For this review, take the finished solid that the model builds, in its own axes (mm). Face numbers are marked on the shaded views. A direction names the side the tool comes from. Coordinates: 2 decimals unless noted, no trailing zeros. Order: outer loops, then holes, each group sorted by start corner. A loop starts at its lowest first (then second) coordinate and runs counter-clockwise, first axis right, second up.
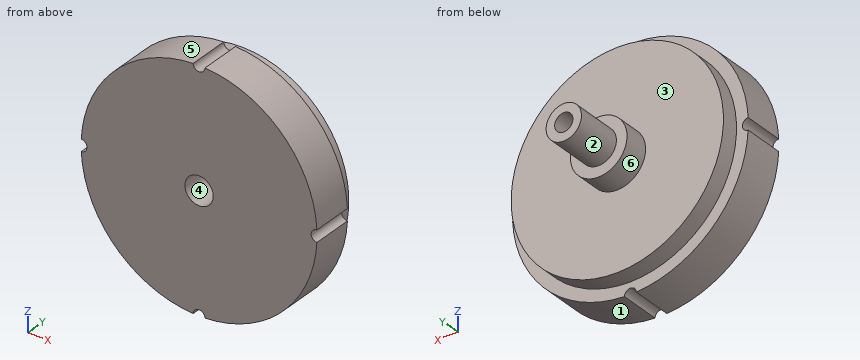
from build123d import *

# Parameters (mm, degrees)
CUT_EXTRUDE1_DEPTH      = 18.993488406
CUT_EXTRUDE1_DEPTH_BACK = 18.993488406
SKETCH5_R               = 0.5


with BuildPart() as part:
    # Sketch4 → Revolve1 (revolve)
    with BuildSketch(Plane.XY, mode=Mode.PRIVATE) as revolve1_sk:
        Polygon((-0.775, 11.125), (-0.775, 4), (-1.2, 4), (-1.2, 0), (-10, 0), (-10, 3.5), (-9, 3.5), (-9, 5), (-2.4, 5), (-2.4, 7.125), (-1.5, 7.125), (-1.5, 11.125), align=None)
    revolve(revolve1_sk.sketch.rotate(Axis((0, 0, 0), (0, 1, 0)), 270), axis=Axis((0, 0, 0), (0, 1, 0)))

    # Sketch5 → Cut-Extrude1 (cut, two sides: drawn at the far end of the back side and taken through both)
    with BuildSketch(Plane.XZ.offset(-CUT_EXTRUDE1_DEPTH_BACK)):
        with Locations((0, 10)):
            Circle(SKETCH5_R)
        with Locations((10, 0)):
            Circle(SKETCH5_R)
        with Locations((0, -10)):
            Circle(SKETCH5_R)
        with Locations((-10, 0)):
            Circle(SKETCH5_R)
    extrude(amount=CUT_EXTRUDE1_DEPTH + CUT_EXTRUDE1_DEPTH_BACK, mode=Mode.SUBTRACT)


solid = part.part
1. Take a section at D-D, the plane x = -6.5. Give the boundary of the cut face in (y, z).
Answer below:
outline: (0, -7.6) - (3.5, -7.6) - (3.5, -6.22) - (5, -6.22) - (5, 6.22) - (3.5, 6.22) - (3.5, 7.6) - (0, 7.6) - close
2. The part is to be moulded in two halves that separate along X. For the marked faces 1, 2, 3 and 4, say which applies: +X half, -X half, draft (parallel to the pull), parting line (faces both ways), or undercut.
Answer below:
face 1: +X half
face 2: parting line
face 3: draft
face 4: undercut
3. To check wall thickness, follow L1, parallel to Y at x = 1.25, z = -5; L2, parallel to Z at x = 0.25, y = 6.25; L3, parallel to Z at x = 6.75, y = 4.25. State the ranges of each line that lie inside material, in increasing order.
Answer below:
L1: y = 0 to 5
L2: z = -2.39 to -0.73, 0.73 to 2.39
L3: z = -5.95 to 5.95
4. Take a section at B-B, the plane x = 0. Give the boundary of the cut face in (y, z) (3 decimals), plus the area to 3 significant figures.
Answer below:
outline: (0, -9.5) - (3.5, -9.5) - (3.5, -9) - (5, -9) - (5, -2.4) - (7.125, -2.4) - (7.125, -1.5) - (11.125, -1.5) - (11.125, -0.775) - (4, -0.775) - (4, -1.2) - (0, -1.2) - close; (0, 1.2) - (4, 1.2) - (4, 0.775) - (11.125, 0.775) - (11.125, 1.5) - (7.125, 1.5) - (7.125, 2.4) - (5, 2.4) - (5, 9) - (3.5, 9) - (3.5, 9.5) - (0, 9.5) - close
area: 95.1 mm2
5. Clearance check with flat-ended pins moving along their axes: pin 1 Ø10 at (x, z) = (1.5, 1) entering from +Y (3 decimals); pin 2 Ø2 at (x, y) = (4, 2) entering from -Z; pin 3 Ø2 at (x, z) = (0, 0) entering from -Y; pin 4 Ø2 at (x, y) = (-2, 9) entering from -Z. State where each tip first meets the part, or that it passes through.
Answer below:
pin 1: stops at y = 11.125
pin 2: stops at z = -9.54
pin 3: stops at y = 4
pin 4: stops at z = -1.12
6. Machinability: for the marked faces 5 and 6, which of the approach directions +Z, -Z, +X, -X, +Y, -Y give a long, thin tool a straight path to every point of the face, cutting with its end or side? Answer none if there is none.
Answer below:
face 5: +Z, -X, +Y, -Y
face 6: +Y
7. Take a section at A-A, the plane z = 0. Give the boundary of the cut face in (x, y) (3 decimals), plus the area to 3 significant figures.
Answer below:
outline: (-9.5, 0) - (-1.2, 0) - (-1.2, 4) - (-0.775, 4) - (-0.775, 11.125) - (-1.5, 11.125) - (-1.5, 7.125) - (-2.4, 7.125) - (-2.4, 5) - (-9, 5) - (-9, 3.5) - (-9.5, 3.5) - close; (0.775, 4) - (1.2, 4) - (1.2, 0) - (9.5, 0) - (9.5, 3.5) - (9, 3.5) - (9, 5) - (2.4, 5) - (2.4, 7.125) - (1.5, 7.125) - (1.5, 11.125) - (0.775, 11.125) - close
area: 95.1 mm2
8. Take a section at C-C, the plane y = 10.5. Give the boundary of the cut face in (x, z) (3 decimals).
Answer below:
outline: circle Ø3 at (0, 0); hole circle Ø1.55 at (0, 0)
